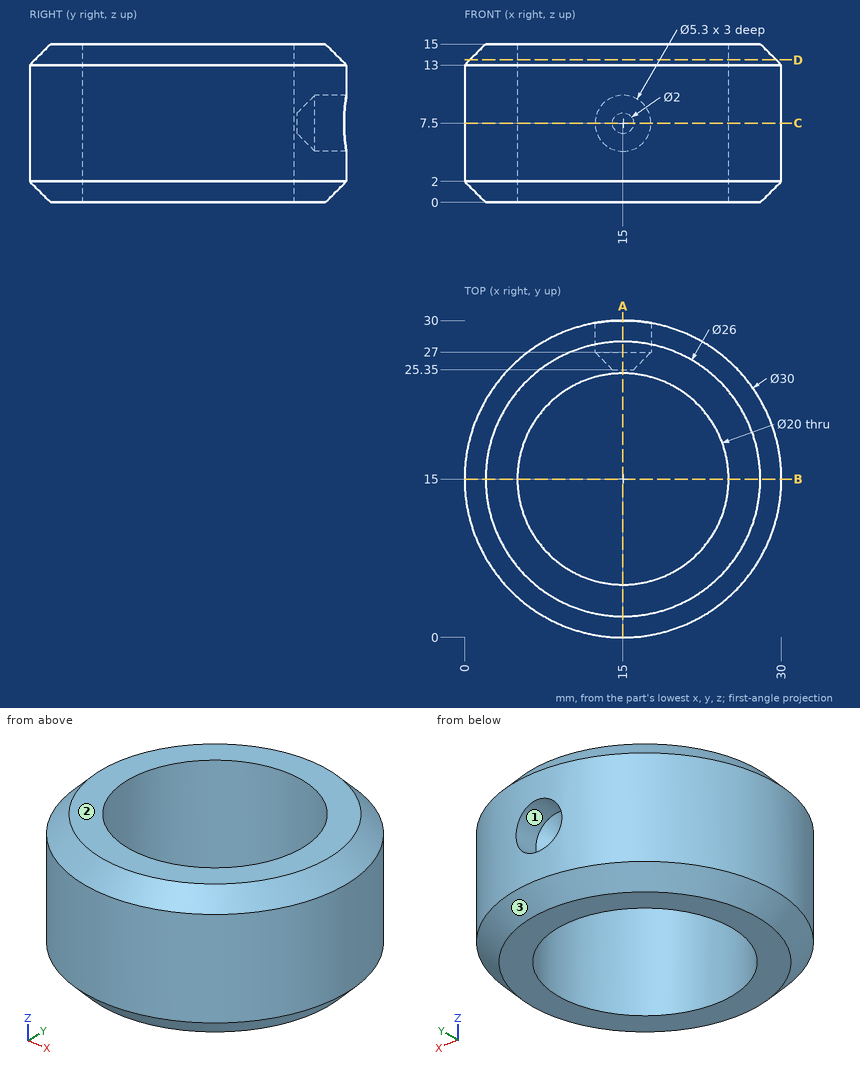
Geometry check sheet. Reference: drawing and pictorial views, mm from the part's lowest x, y, z. Round coordinates to 2 decimals unless told otherwise and drop trailing zeros. Loops run counter-clockwise (first coordinate to the right, second up) from the corner with the lowest first, then second, coordinate; pieces in that order, holes last. Notation, with made-up numbers: (82.25, 8) - (112.25, 8) arc R7 ccw to (112.25, 13) - close; hole circle Ø7 at (40, -12). An arc over 180 degrees is marked (long way). Use a Markdown table: item, result.
Q1. Draft check along X on the marked faces 1, 2 and 3. Enter one of: released by +X, released by -X, zero draft, split by the parting line, or undercut.
Solutions:
| item | result |
|---|---|
| face 1 | undercut |
| face 2 | zero draft |
| face 3 | split by the parting line |
Q2. Go/stop test with flat-tipped pins: P1, Ø8, axis at y = 10.5, z = 2, coming from the +X side; P2, Ø12, axis at x = 10.5, y = 20, coming from the +Z side; P3, Ø3, axis at x = 6.5, z = 11, coming from the +Y side; P4, Ø5, axis at x = 15, z = 7.5, coming from the +Y side. Record where each tip stops, or that it passes through.
Solutions:
| item | result |
|---|---|
| P1 | stops at x = 29.99 |
| P2 | stops at z = 15 |
| P3 | stops at y = 28.27 |
| P4 | stops at y = 26.85 |
Q3. Cross-section at B-B on y = 15. Record the cut outline in (x, z).
Solutions:
| item | result |
|---|---|
| outline | (0, 2) - (2, 0) - (5, 0) - (5, 15) - (2, 15) - (0, 13) - close; (25, 0) - (28, 0) - (30, 2) - (30, 13) - (28, 15) - (25, 15) - close |
Q4. Material ranges on line 1 (Y direction, x = 15, z = 11.75); line 2 (Y direction, x = 15, z = 7); line 3 (X direction, y = 27.75, z = 7.5), recorded low to high.
Solutions:
| item | result |
|---|---|
| line 1 | y = 0 to 5, 25 to 30 |
| line 2 | y = 0 to 5, 25 to 25.35 |
| line 3 | x = 7.1 to 12.35, 17.65 to 22.9 |
Q5. Cross-section at D-D on z = 13.5. Record the cut outline in (x, y).
Solutions:
| item | result |
|---|---|
| outline | circle Ø29 at (15, 15); hole circle Ø20 at (15, 15) |
Q6. Cross-section at C-C on z = 7.5. Record the cut outline in (x, y).
Solutions:
| item | result |
|---|---|
| outline | (12.35, 27) - (12.35, 29.76) arc R15 ccw (long way) to (17.65, 29.76) - (17.65, 27) - (16, 25.35) - (14, 25.35) - close; hole circle Ø20 at (15, 15) |
Q7. Cross-section at A-A on x = 15. Record the cut outline in (y, z), plus the area to 3 significant figures.
Solutions:
| item | result |
|---|---|
| outline | (0, 2) - (2, 0) - (5, 0) - (5, 15) - (2, 15) - (0, 13) - close; (25, 0) - (28, 0) - (30, 2) - (30, 4.85) - (27, 4.85) - (25.35, 6.5) - (25.35, 8.5) - (27, 10.15) - (30, 10.15) - (30, 13) - (28, 15) - (25, 15) - close |
| area | 120 mm2 |
